Solid Edge part; units mm, degrees
sketch "Sketch1" plane through (0, 0, 0) normal (1, 0, 0) x (0, 1, 0)
  line L0 (9.9137, 19.9194) -> (48.1572, 0.886)
  arc A0 (48.1572, 0.886) -> (44.5928, -6.276) centre (46.375, -2.695) cw
  line L1 (6.3492, 12.7574) -> (44.5928, -6.276)
  arc A1 (-7.125, 12.3409) -> (6.3492, 12.7574) centre (0, 0) cw
  arc A2 (-7.125, 12.3409) -> (-11.125, 19.2691) centre (-9.125, 15.805) cw
  arc A3 (-11.125, 19.2691) -> (9.9137, 19.9194) centre (0, 0) cw
  circle A4 centre (46.375, -2.695) radius 1.45
  circle A5 centre (-9.125, 15.805) radius 2.2
extrude "Protrusion1" add sketch "Sketch1" along normal blind 2
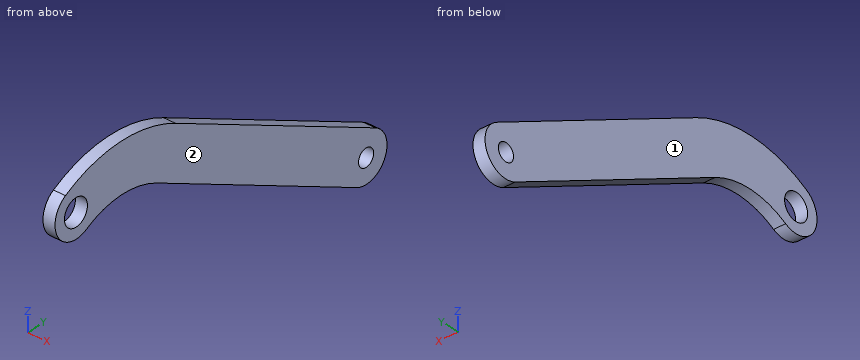
Input: part model. Units: mm. Frame: model coordinates. Face numbers are marked on the shaded views. Give positions to 0.01 mm unless a question says otherwise; leave off trailing zeros. Write each loop counter-clockwise with the first axis right and the second up, starting at its lowest first coordinate (ties: lowest second). Pieces come first, ordered by that corner, then holes.
Q1. Section A-A, the plane x = 1.55. Output: boundary loops of the cut face in (y, z) (3 decimals), plus the area to 3 significant figures.
Q2. First-contact query: P1, Ø6, axis at y = 5, z = 7, coming from the -X side. Flat tip, straight axial feed; report the tip coordinate or a pass-through.
Q3. Section C-C, the plane y = 20. Output: boundary loops of the cut face in (x, z).
Q4. Material intervals for probe 1 along Y at (x, z) = (1, -2.5); probe 2 along Y at (x, z) = (1.7, -3); probe 3 along Z at (x, y) = (1, 0), sorted ascending.
Q5. Pull-direction query (X, two-part tool) for the marked faces 1 and 2; classes: pulls with the +X half, pulls with the -X half, needs draft (parallel to the pull), parting line crosses it, or undercut.
Q6. Section B-B, the plane z = -2. Output: boundary loops of the cut face in (x, y), plus the area to 3 significant figures.
Filled in:
1. outline: (-11.125, 19.269) arc R4 ccw to (-7.125, 12.341) arc R14.25 cw to (6.349, 12.757) - (44.593, -6.276) arc R4 ccw to (48.157, 0.886) - (9.914, 19.919) arc R22.25 ccw to start; hole circle Ø4.4 at (-9.125, 15.805); hole circle Ø2.9 at (46.375, -2.695)
1. area: 514 mm2
2. P1: passes through
3. outline: (0, 5.96) - (2, 5.96) - (2, 14.9) - (0, 14.9) - close
4. probe 1: y = 37.01 to 44.94, 47.81 to 50.37
4. probe 2: y = 38.01 to 44.96, 47.79 to 50.36
4. probe 3: z = 14.25 to 22.25
5. face 1: pulls with the -X half
5. face 2: pulls with the +X half
6. outline: (0, 36) - (2, 36) - (2, 45.1) - (0, 45.1) - close; (0, 47.65) - (2, 47.65) - (2, 50.31) - (0, 50.31) - close
6. area: 23.5 mm2
